Verification items for the finished model (mm, model axes). Face numbers are marked on the shaded views. Round coordinates to 2 decimals unless told otherwise and drop trailing zeros. Write each loop counter-clockwise with the first axis right and the second up, starting at its lowest first coordinate (ties: lowest second). Pieces come first, ordered by that corner, then holes. Notation, with made-up numbers: M -29,-14.5 L -21,-14.5 A33 cw -21,14.5 Z; hole C 11.5,-22 d3. An arc over 180 degrees is marked long. One line per item, written item: value. Start each with the question number.
Item 1: Section check B-B, the plane y = 1.4. State how many separate pieces and enclosed holes the cut face has, then the cut area to 3 significant figures.
Item 2: Section check C-C, the plane z = 1.5. Record the cut outline in (x, y).
Item 3: Draft check along Z on the marked faces 1, 2 and 3. Enter one of: +Z half, -Z half, draft (parallel to the pull), parting line (faces both ways), or undercut.
Item 4: Section check A-A, the plane x = 0. Record the cut outline in (y, z), then the cut area to 3 significant figures.
Item 5: Gauge pin test, flat end, axial feed: pin 1 (1 mm diameter, centred on y = 0.5, z = -0.5, fed in from -X). Record the tip position at first contact, or that the pin passes through.
Item 6: Thickness scan on probe 1 along Z at (x, y) = (16.16, 1); probe 2 along X at (y, z) = (0.65, 1.25); probe 3 along X at (y, z) = (1.25, 1.75). Record the ranges inside material, lowest first. Write a range as from..to.
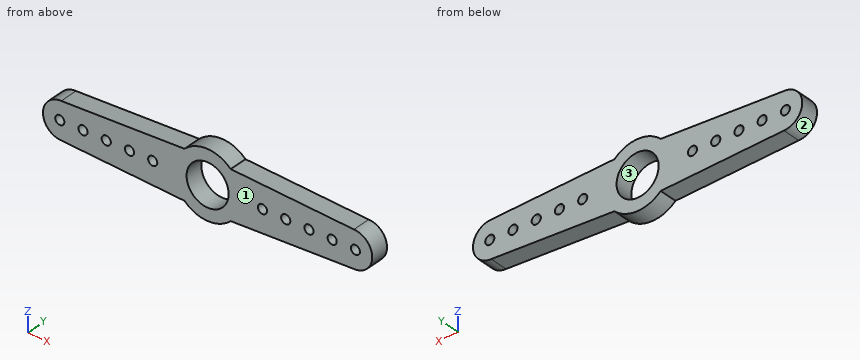
from build123d import *

# Parameters (mm, degrees)
SKETCH1_R           = 2.3
SKETCH1_R_2         = 0.5
BOSS_EXTRUDE1_DEPTH = 2


with BuildPart() as part:
    # Sketch1 → Boss-Extrude1 (new body)
    with BuildSketch(Plane(origin=(0, 0, 0), x_dir=(1, 0, 0), z_dir=(0, 1, 0))):
        with BuildLine():
            Line((-16, -2), (-2.528486514, -2.632548127))
            ThreePointArc((-2.528486514, -2.632548127), (1e-09, -3.650200137), (2.528486517, -2.632548127))
            Line((2.528486517, -2.632548127), (16, -2))
            ThreePointArc((16, -2), (18, 0), (16, 2))
            Line((16, 2), (2.528048307, 2.632568703))
            ThreePointArc((2.528048307, 2.632568703), (1e-09, 3.649799863), (-2.528048304, 2.632568703))
            Line((-2.528048304, 2.632568703), (-16, 2))
            ThreePointArc((-16, 2), (-18, 0), (-16, -2))
        make_face()
        with Locations(Location((0, 0, 0), (0, 0, 270))):
            Circle(SKETCH1_R, mode=Mode.SUBTRACT)
        with Locations(Location((-6, 0, 0), (0, 0, 270))):
            Circle(SKETCH1_R_2, mode=Mode.SUBTRACT)
        with Locations(Location((-8.54, 0, 0), (0, 0, 270))):
            Circle(SKETCH1_R_2, mode=Mode.SUBTRACT)
        with Locations(Location((-11.08, 0, 0), (0, 0, 270))):
            Circle(SKETCH1_R_2, mode=Mode.SUBTRACT)
        with Locations(Location((-13.62, 0, 0), (0, 0, 270))):
            Circle(SKETCH1_R_2, mode=Mode.SUBTRACT)
        with Locations(Location((-16.16, 0, 0), (0, 0, 270))):
            Circle(SKETCH1_R_2, mode=Mode.SUBTRACT)
        with Locations(Location((16.16, 0, 0), (0, 0, 90))):
            Circle(SKETCH1_R_2, mode=Mode.SUBTRACT)
        with Locations(Location((13.62, 0, 0), (0, 0, 90))):
            Circle(SKETCH1_R_2, mode=Mode.SUBTRACT)
        with Locations(Location((11.08, 0, 0), (0, 0, 90))):
            Circle(SKETCH1_R_2, mode=Mode.SUBTRACT)
        with Locations(Location((8.54, 0, 0), (0, 0, 90))):
            Circle(SKETCH1_R_2, mode=Mode.SUBTRACT)
        with Locations(Location((6, 0, 0), (0, 0, 90))):
            Circle(SKETCH1_R_2, mode=Mode.SUBTRACT)
    extrude(amount=BOSS_EXTRUDE1_DEPTH)


solid = part.part
Response values:
1. separate pieces: 1
1. enclosed holes: 11
1. area: 147 mm2
2. outline: M -17.32,0 L -1.74,0 L -1.74,2 L -17.32,2 Z; M 1.74,0 L 17.32,0 L 17.32,2 L 1.74,2 Z
3. face 1: draft
3. face 2: parting line
3. face 3: undercut
4. outline: M 0,-3.65 L 2,-3.65 L 2,-2.3 L 0,-2.3 Z; M 0,2.3 L 2,2.3 L 2,3.65 L 0,3.65 Z
4. area: 5.40 mm2
5. pin 1: stops at x = -18
6. probe 1: z = -1.99..-0.5, 0.5..1.99
6. probe 2: x = -17.56..-1.93, 1.93..17.56
6. probe 3: x = -16.97..-1.49, 1.49..16.97
